from build123d import *

# Parameters (mm, degrees)
SKETCH1_W           = 114.3
SKETCH1_H           = 114.3
BOSS_EXTRUDE1_DEPTH = 25.4
CHAMFER1_SIZE       = 12.7
SKETCH2_R           = 6.35
CUT_EXTRUDE1_DEPTH  = 5.08


with BuildPart() as part:
    # Sketch1 → Boss-Extrude1 (new body)
    with BuildSketch(Plane(origin=(0, 0, 0), x_dir=(1, 0, 0), z_dir=(0, 1, 0))):
        Rectangle(SKETCH1_W, SKETCH1_H)
    extrude(amount=BOSS_EXTRUDE1_DEPTH)

    # Chamfer1
    chamfer1_edges = [part.edges().sort_by_distance(p)[0] for p in [
        (57.15, 12.7, 57.15),
        (-57.15, 12.7, 57.15),
        (-57.15, 12.7, -57.15),
        (57.15, 12.7, -57.15),
    ]]
    chamfer(chamfer1_edges, length=CHAMFER1_SIZE)

    # Sketch2 → Cut-Extrude1 (cut)
    with BuildSketch(Plane(origin=(0, 0, 0), x_dir=(-1, 0, 0), z_dir=(0, -1, 0))):
        with Locations(Location((0, -47.625, 0), (0, 0, 90))):
            Circle(SKETCH2_R)
    extrude(amount=-CUT_EXTRUDE1_DEPTH, mode=Mode.SUBTRACT)


solid = part.part
Source: CAD feature listing. Evaluate the final solid. Frame: model axes, mm. A direction names the side the tool comes from. Round coordinates to 2 decimals unless told otherwise and drop trailing zeros. Loops run counter-clockwise (first coordinate to the right, second up) from the corner with the lowest first, then second, coordinate; pieces in that order, holes last. Notation, with made-up numbers: (9.5, 35) - (21.5, 35) arc R30 ccw to (21.5, 71) - close; hole circle Ø2 at (17, 8.5). An arc over 180 degrees is marked (long way). Write item = value, one per line. Start each with the question number.
Item 1: Section query B-B on x = 0. Output: boundary loops of the cut face in (y, z) (3 decimals), plus the area to 3 significant figures.
Item 2: Section query A-A on y = 2.25. Output: boundary loops of the cut face in (x, z) (3 decimals), plus the area to 3 significant figures.
Item 3: Section query D-D on x = 46.5. Output: boundary loops of the cut face in (y, z), plus the area to 3 significant figures.
Item 4: Material intervals for line 1 (Y direction, x = -1, z = 46.5); line 2 (Z direction, x = -52, y = 15.5); line 3 (Z direction, x = -51.5, y = 16), sorted ascending.
Item 5: First-contact query: pin 1 Ø20.5 at (x, z) = (0, 47.625) entering from -Y; pin 2 Ø6.5 at (x, z) = (-2, 48) entering from -Y. Flat tips, straight axial feed; report the tip coordinate or a pass-through.
Item 6: Section query C-C on y = 10.5. Output: boundary loops of the cut face in (x, z), plus the area to 3 significant figures.
Item 7: Mould query, pull axis Z, two halves, no side actions, for faces 1 (the face through (0.28, 2.5, 53.97)), 2 (the face through (-50.7, 12.5, 50.9)), 3 (the face through (-50.7, 12.5, -50.9)). Classes: released by +Z, released by -Z, zero draft, split by the parting line, or undercut.
Item 8: Reachability of faces 4 (the face through (-1, 13, 57.15)), 5 (the face through (0, 5.08, 48)) from +Z, -Z, +X, -X, +Y, -Y: full face, straight path, thin tool, end or side. Return the list, or none.
Results list:
q1.outline = (0, -57.15) - (25.4, -57.15) - (25.4, 57.15) - (0, 57.15) - (0, 53.975) - (5.08, 53.975) - (5.08, 41.275) - (0, 41.275) - close
q1.area = 2,840 mm²
q2.outline = (-57.15, -44.45) - (-44.45, -57.15) - (44.45, -57.15) - (57.15, -44.45) - (57.15, 44.45) - (44.45, 57.15) - (-44.45, 57.15) - (-57.15, 44.45) - close; hole circle Ø12.7 at (0, 47.625)
q2.area = 12,600 mm²
q3.outline = (0, -55.1) - (25.4, -55.1) - (25.4, 55.1) - (0, 55.1) - close
q3.area = 2,800 mm²
q4.line_1 = 5.08 to 25.4
q4.line_2 = -49.6 to 49.6
q4.line_3 = -50.1 to 50.1
q5.pin_1 = 0
q5.pin_2 = 5.08
q6.outline = (-57.15, -44.45) - (-44.45, -57.15) - (44.45, -57.15) - (57.15, -44.45) - (57.15, 44.45) - (44.45, 57.15) - (-44.45, 57.15) - (-57.15, 44.45) - close
q6.area = 12,700 mm²
q7.face_1 = undercut
q7.face_2 = released by +Z
q7.face_3 = released by -Z
q8.face_4 = +Z, +X, -X, +Y, -Y
q8.face_5 = -Y
